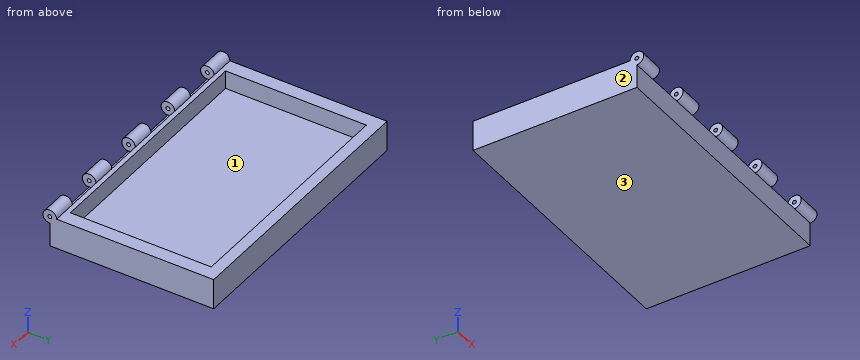
```python
from build123d import *

# Parameters (mm, degrees)
SKETCH_W            = 220
SKETCH_H            = 135
PAD_DEPTH           = 25
SKETCH001_W         = 197
SKETCH001_H         = 116
POCKET_DEPTH        = 15
SKETCH002_R         = 5.5
POCKET001_DEPTH     = 220.001
SKETCH004_R         = 5.6
PAD001_DEPTH        = 20
LINEARPATTERN_COUNT = 5
LINEARPATTERN_PITCH = 50
SKETCH005_R         = 1.6
POCKET002_DEPTH     = 220.001


with BuildPart() as part:
    # Sketch → Pad (new body)
    with BuildSketch(Plane.XY):
        Rectangle(SKETCH_W, SKETCH_H)
    extrude(amount=PAD_DEPTH)

    # Sketch001 (on Face6 of Pad) → Pocket (cut)
    with BuildSketch(Plane.XY.offset(25)):
        Rectangle(SKETCH001_W, SKETCH001_H)
    extrude(amount=-POCKET_DEPTH, mode=Mode.SUBTRACT)

    # Sketch002 (on Face3 of Pocket) → Pocket001 (cut, through all)
    with BuildSketch(Plane.YZ.offset(110)):
        with Locations((-67.5, 25)):
            Circle(SKETCH002_R)
    extrude(amount=-POCKET001_DEPTH, mode=Mode.SUBTRACT)

    # Sketch004 (on Face3 of Pocket001) → Pad001 (join)
    with BuildSketch(Plane.YZ.offset(110)):
        with Locations((-67.5, 25)):
            Circle(SKETCH004_R)
    pad001 = extrude(amount=-PAD001_DEPTH)

    # LinearPattern: Pad001 ×5
    with Locations(*[(-i * LINEARPATTERN_PITCH, 0, 0) for i in range(1, LINEARPATTERN_COUNT)]):
        add(pad001)

    # Sketch005 (on Face31 of LinearPattern) → Pocket002 (cut, through all)
    with BuildSketch(Plane.YZ.offset(110)):
        with Locations((-67.5, 25)):
            Circle(SKETCH005_R)
    extrude(amount=-POCKET002_DEPTH, mode=Mode.SUBTRACT)


solid = part.part
```
Geometry check sheet. Reference: the model listing, model coordinates, mm. Face numbers are marked on the shaded views. Round coordinates to 2 decimals unless told otherwise and drop trailing zeros. Order: outer loops, then holes, each group sorted by start corner. A loop starts at its lowest first (then second) coordinate and runs counter-clockwise, first axis right, second up. Notation, with made-up numbers: M 52,-34.5 L 104,-34.5 A25 cw 104,-8.5 Z; hole C -18,23 d2. An arc over 180 degrees is marked long. Answer as CSV lines item,"result".
1) Mould release check, pull along X, two halves, no side actions. Record for the marked faces 1, 2 and 3: +X half, -X half, draft (parallel to the pull), parting line (faces both ways), or undercut.
Entries:
face 1,"undercut"
face 2,"-X half"
face 3,"draft"
2) Sectioned sample at D-D on z = 3. Record the cut outline in (x, y), and give its area (3 significant figures).
Entries:
outline,"M -110,-67.5 L 110,-67.5 L 110,67.5 L -110,67.5 Z"
area,"29,700 mm2"
3) Gauge pin test, flat ends, axial feed: pin 1 Ø8 at (x, y) = (72, 45) entering from +Z; pin 2 Ø8 at (x, y) = (-7, 43.5) entering from -Z; pin 3 Ø3 at (x, z) = (6.5, 18.5) entering from -Y; pin 4 Ø6 at (x, z) = (-17.5, 5) entering from -Y. Record the tip position at first contact, or that the pin passes through.
Entries:
pin 1,"z = 10"
pin 2,"z = 0"
pin 3,"y = -70.02"
pin 4,"y = -67.5"
4) Thickness scan on probe 1 along X at (y, z) = (-32, 17.5); probe 2 along Y at (x, z) = (-9, 17); probe 3 along Z at (x, y) = (86, 13). Record the ranges inside material, lowest first. Write a range as [from, to].
Entries:
probe 1,"[-110, -98.5], [98.5, 110]"
probe 2,"[-67.5, -58], [58, 67.5]"
probe 3,"[0, 10]"
5) Sectioned sample at C-C on y = -31. Record the cut outline in (x, z).
Entries:
outline,"M -110,0 L 110,0 L 110,25 L 98.5,25 L 98.5,10 L -98.5,10 L -98.5,25 L -110,25 Z"
6) Sectioned sample at B-B on x = -51.5. Record the cut outline in (y, z), and give its area (3 significant figures).
Entries:
outline,"M -67.5,0 L 67.5,0 L 67.5,25 L 58,25 L 58,10 L -58,10 L -58,25 L -61.9,25 A5.6 ccw long -67.5,19.4 Z; hole C -67.5,25 d3.2"
area,"1,700 mm2"
7) Sectioned sample at A-A on z = 17. Record the cut outline in (x, y).
Entries:
outline,"M -110,-67.5 L 110,-67.5 L 110,67.5 L -110,67.5 Z; hole M -98.5,-58 L 98.5,-58 L 98.5,58 L -98.5,58 Z"
